Can you work these out from the drawing? Everything is in mm from the part's minimum corner. Round coordinates to 2 decimals unless told otherwise and drop trailing zeros. Order: outer loops, then holes, each group sorted by start corner. A loop starts at its lowest first (then second) coordinate and runs counter-clockwise, first axis right, second up. Notation, with made-up numbers: (62.25, -30.5) -> (107.25, -30.5) arc R27 ccw to (107.25, -11.5) -> close; hole circle Ø6 at (62, 9). An arc over 180 degrees is marked (long way). One line per item, written item: value.
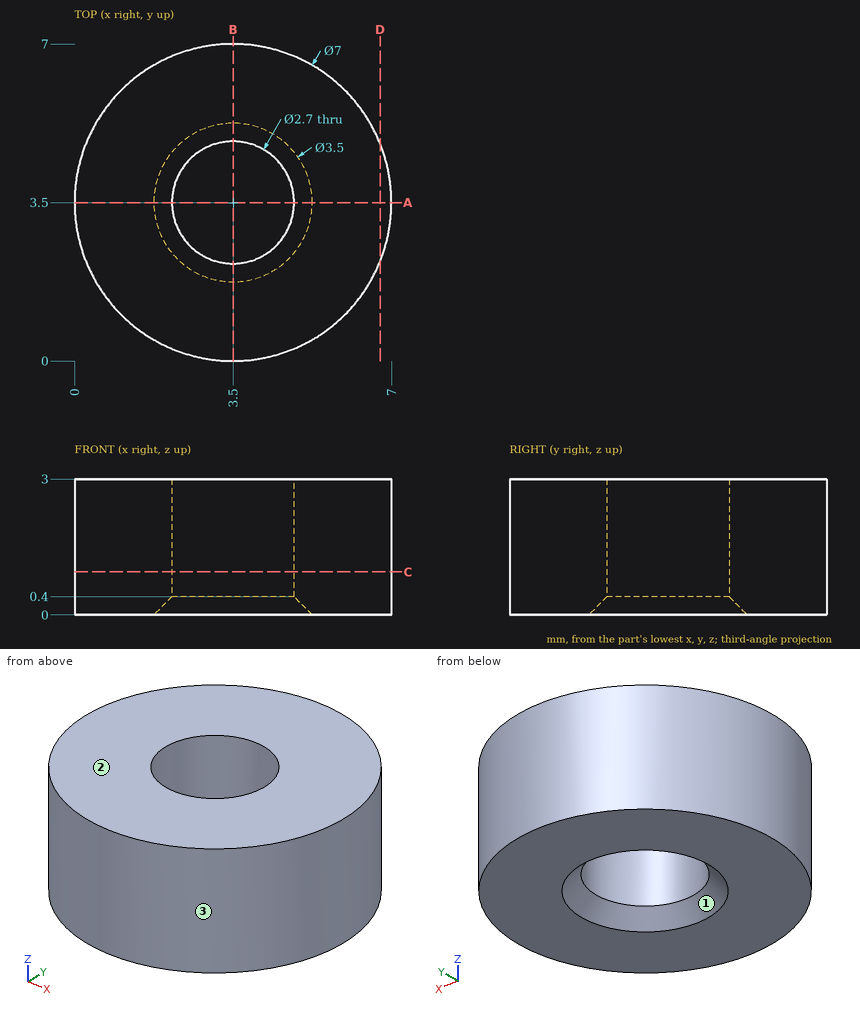
Q1. I want a section at D-D on x = 6.75. List the corners of the cut face in (y, z) for me, plus the area to 3 significant figures.
Answers below:
outline: (2.2, 0) -> (4.8, 0) -> (4.8, 3) -> (2.2, 3) -> close
area: 7.79 mm^2
Q2. I want a section at A-A on y = 3.5. List the corners of the cut face in (x, z) for me, plus the area to 3 significant figures.
Answers below:
outline: (0, 0) -> (1.75, 0) -> (2.15, 0.4) -> (2.15, 3) -> (0, 3) -> close; (4.85, 0.4) -> (5.25, 0) -> (7, 0) -> (7, 3) -> (4.85, 3) -> close
area: 12.7 mm^2
Q3. Please list where these lines run through material, in increasing order: line 1 along Y through (x, z) = (3.5, 1); line 2 along X through (y, z) = (4, 0.7); line 3 along Y through (x, z) = (4.5, 1.8).
Answers below:
line 1: 0 to 2.15, 4.85 to 7
line 2: 0.04 to 2.25, 4.75 to 6.96
line 3: 0.15 to 2.59, 4.41 to 6.85
Q4. Will these pins go through, and if not, where does the flat tip stop? pin 1 Ø1 at (y, z) = (5.5, 2.5) entering from -X; pin 2 Ø1.5 at (x, z) = (5.5, 2) entering from +Y.
Answers below:
pin 1: x = 0.34
pin 2: y = 6.77
Q5. We'd pull the mould along X, two halves only. Please class the marked faces 1, 2 and 3: released by +X, released by -X, zero draft, split by the parting line, or undercut.
Answers below:
face 1: undercut
face 2: zero draft
face 3: split by the parting line
Q6. I want a section at C-C on z = 0.95. List the corners of the cut face in (x, y) for me.
Answers below:
outline: circle Ø7 at (3.5, 3.5); hole circle Ø2.7 at (3.5, 3.5)
